Part model, mm, in its own coordinate system. Round coordinates to 2 decimals unless told otherwise and drop trailing zeros. Loops run counter-clockwise (first coordinate to the right, second up) from the corner with the lowest first, then second, coordinate; pieces in that order, holes last. Notation, with made-up numbers: M 12,18 L 51,18 A19 ccw 51,31 Z; hole C 59.25,79 d3. An arc over 180 degrees is marked long. Put each result on its own line as item: value. Start each with the question number.
1) Slice it at D-D on z = -105.5. Give the cut face in (x, y).
2) Slice it at C-C on y = 0.55. State how many separate pieces and enclosed holes the cut face has, then the cut area to 3 significant figures.
3) Slice it at A-A on z = -20. Give the cut face in (x, y), then the cut area to 3 significant figures.
4) Slice it at B-B on x = -9. Give the cut face in (y, z), then the cut area to 3 significant figures.
5) Probe line 1 along Z through (x, y) = (-12, 2.85); line 2 along Z through (x, y) = (28, 2.2); line 3 along X through (y, z) = (1.8, 49). List the from-to ranges inside material, lowest first.
6) Drop flat-ended pins along their axis: pin 1 Ø1.5 at (y, z) = (1, 118.5) entering from -X; pin 2 Ø0.9 at (x, y) = (-26, 2) entering from +Z; pin 3 Ø1.5 at (x, y) = (-26.5, 1.5) entering from -Z. Give the stop position or say it passes through.
Autodesk Inventor part; units mm, degrees
ref_plane "YZ Plane" through (0, 0, 0) normal (1, 0, 0) x (0, 1, 0)
ref_plane "XZ Plane" through (0, 0, 0) normal (0, 1, 0) x (-1, 0, 0)
ref_plane "XY Plane" through (0, 0, 0) normal (0, 0, 1) x (1, 0, 0)
sketch "Sketch1" plane through (0, 0, 0) normal (0, 1, 0) x (-1, 0, 0)
  line L0 (-25, 190) -> (25, 190)
  line L1 (25, 190) -> (25, -190)
  line L2 (25, -190) -> (-25, -190)
  line L3 (-25, -190) -> (-25, 190)
  line L4 (-25, 190) -> (25, -190) construction
  line L5 (25, 190) -> (-25, -190) construction
  point P0 (0, 0)
  dimension "d0" = 50
  dimension "d1" = 380
extrude "Extrusion1" add sketch "Sketch1" along normal blind 3
sketch "Sketch2" plane through (0, 3, 0) normal (0, 1, 0) x (1, 0, 0)
  line L0 (25, -160) -> (50, -160)
  line L1 (50, -160) -> (50, -120)
  line L2 (50, -120) -> (25, -120)
  line L3 (25, -120) -> (25, -160)
  line L4 (50, -40) -> (20, -40)
  line L5 (20, -40) -> (20, 40)
  line L6 (20, 40) -> (50, 40)
  line L7 (50, 40) -> (50, -40)
  line L8 (50, -40) -> (20, 40) construction
  line L9 (20, -40) -> (50, 40) construction
  line L10 (30, 160) -> (50, 160)
  line L11 (50, 160) -> (50, 120)
  line L12 (50, 120) -> (30, 120)
  line L13 (30, 120) -> (30, 160)
  circle A0 centre (50, -140) radius 20
  circle A1 centre (50, -20) radius 20
  circle A2 centre (50, 20) radius 20
  circle A3 centre (50, 140) radius 20
  line L14 (25, 190) -> (25, -190)
  line L15 (25, -190) -> (25, 190)
  line L16 (30, 160) -> (25, 160)
  line L17 (25, 160) -> (25, 120)
  line L18 (25, 120) -> (30, 120)
  line L19 (30, 120) -> (30, 160)
  line L20 (25, -120) -> (25, -120)
  line L21 (25, -120) -> (25, -150)
  line L22 (25, -150) -> (25, -150)
  line L23 (25, -150) -> (25, -120)
  line L24 (50, 0) -> (35, 0)
  line L25 (35, 0) -> (35, 5)
  line L26 (35, 5) -> (50, 5)
  line L27 (50, 5) -> (50, 0)
  line L28 (25, 190) -> (-25, 190)
  line L29 (-25, -190) -> (25, -190)
  point P0 (0, 0)
  point P1 (35, 0)
  dimension "d10" = 40
  dimension "d4" = 25
  dimension "d5" = 40
  dimension "d7" = 80
  dimension "d8" = 20
  dimension "d9" = 40
  dimension "d11" = 40
  dimension "d12" = 20
  dimension "d13" = 20
  dimension "d16" = 80
  dimension "d17" = 80
  dimension "d18" = 5
  dimension "d19" = 25
  dimension "d20" = 25
  dimension "d40" = 15
  dimension "d41" = 30
  dimension "d43" = 70
  dimension "d44" = 40
  dimension "d49" = 70
extrude "Extrusion2" add sketch "Sketch2" against normal blind 3
sketch "Sketch3" plane through (0, 3, 0) normal (0, 1, 0) x (1, 0, 0)
  line L0 (-25, 190) -> (-25, -190)
  line L1 (-25, -167.5) -> (0, -167.5)
  line L2 (0, -167.5) -> (0, -171.5)
  line L3 (0, -171.5) -> (-25, -171.5)
  line L4 (-25, -171.5) -> (-25, -167.5)
  line L5 (25, -190) -> (-25, -190)
  line L6 (-25, 171.5) -> (0, 171.5)
  line L7 (0, 171.5) -> (0, 167.5)
  line L8 (0, 167.5) -> (-25, 167.5)
  line L9 (-25, 167.5) -> (-25, 171.5)
  line L10 (-25, 190) -> (25, 190)
  point P0 (0, 0)
  dimension "d21" = 25
  dimension "d22" = 4
  dimension "d23" = 18.5
  dimension "d26" = 4
  dimension "d27" = 18.5
  dimension "d50" = 25
extrude "Extrusion3" cut sketch "Sketch3" against normal blind 3
sketch "Sketch4" plane through (0, 0, 0) normal (0, -1, 0) x (1, 0, 0)
  circle A0 centre (50, -20) radius 5.15
  arc A1 (50, -40) -> (50, 0) centre (50, -20) ccw
  circle A2 centre (50, 20) radius 5.15
  line L0 (25, 40) -> (50, 40)
  circle A3 centre (50, -140) radius 5.15
  line L1 (50, -120) -> (25, -120)
  arc A4 (50, -160) -> (50, -120) centre (50, -140) ccw
  circle A5 centre (50, 140) radius 5.15
  line L2 (50, 160) -> (25, 160)
  arc A6 (50, 120) -> (50, 160) centre (50, 140) ccw
  point P0 (0, 0)
  point P1 (25, 160)
  point P2 (25, 290)
  dimension "d28" = 10.3
  dimension "d30" = 0
  dimension "d31" = 10.3
  dimension "d33" = 10.3
  dimension "d36" = 10.3
  dimension "d42" = 40
  dimension "d51" = 0
  dimension "d52" = 0
extrude "Extrusion4" cut sketch "Sketch4" against normal blind 10
sketch "Sketch6" plane through (0, 0, 0) normal (0, -1, 0) x (1, 0, 0)
  line L0 (-25, 167.5) -> (-25, -167.5)
  line L1 (-25, 167.5) -> (0, 167.5)
  line L2 (-21, 147.5) -> (-28, 147.5)
  line L3 (-29, 146.5) -> (-29, 128.5)
  line L4 (-28, 127.5) -> (-21, 127.5)
  line L5 (-21, 127.5) -> (-21, 147.5)
  line L6 (-25, -167.5) -> (-25, 167.5)
  line L7 (-21, 147.5) -> (-29, 127.5) construction
  line L8 (-29, 147.5) -> (-21, 127.5) construction
  arc A0 (-28, 147.5) -> (-29, 146.5) centre (-28, 146.5) ccw
  arc A1 (-29, 128.5) -> (-28, 127.5) centre (-28, 128.5) ccw
  point P0 (0, 0)
  point P1 (-25, 137.5)
  dimension "d54" = 8
  dimension "d55" = 20
  dimension "d56" = 1
  dimension "d57" = 20
extrude "Extrusion5" add sketch "Sketch6" against normal blind 3
pattern_linear "Rectangular Pattern1" count 8 spacing 40 along (0, 0, -1) of "Extrusion5"
properties part number "zijiplaaten"
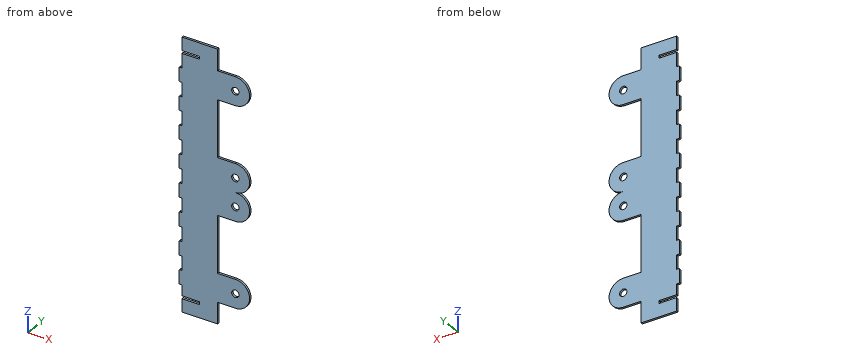
Recorded:
1. outline: M -29,0 L 25,0 L 25,3 L -29,3 Z
2. separate pieces: 1
2. enclosed holes: 4
2. area: 25,600 mm2
3. outline: M -29,0 L 44.85,0 L 44.85,3 L -29,3 Z; M 55.15,0 L 70,0 L 70,3 L 55.15,3 Z
3. area: 266 mm2
4. outline: M 0,-190 L 3,-190 L 3,-171.5 L 0,-171.5 Z; M 0,-167.5 L 3,-167.5 L 3,167.5 L 0,167.5 Z; M 0,171.5 L 3,171.5 L 3,190 L 0,190 Z
4. area: 1,120 mm2
5. line 1: z = -190 to -171.5, -167.5 to 167.5, 171.5 to 190
5. line 2: z = -160 to -120, -40 to 40, 120 to 160
5. line 3: x = -29 to 25
6. pin 1: stops at x = -25
6. pin 2: stops at z = 147.5
6. pin 3: stops at z = -152.5
